The model under review builds one solid part; all positions refer to its coordinate system, in mm. Coordinates: 2 decimals unless noted, no trailing zeros. Order: outer loops, then holes, each group sorted by start corner. A loop starts at its lowest first (then second) coordinate and runs counter-clockwise, first axis right, second up. Notation, with made-up numbers: M 51.25,-6.5 L 81.25,-6.5 A26 ccw 81.25,7.5 Z; hole C -6,-38.75 d10. An arc over 180 degrees is marked long. One line per item, written item: value.
```python
from build123d import *

# Parameters (mm, degrees)
SKETCH1_R           = 5
SKETCH1_R_2         = 1.75
BOSS_EXTRUDE2_DEPTH = 8.5
BOSS_EXTRUDE3_START = -8.5
BOSS_EXTRUDE3_DEPTH = 8.5


with BuildPart() as part:
    # Sketch1 → Boss-Extrude2 (new body)
    # profile 1 of 3: a face of its own
    with BuildSketch(Plane(origin=(0, 0, 0), x_dir=(1, 0, 0), z_dir=(0, 1, 0))):
        Circle(SKETCH1_R)
        with Locations(Location((0, 0, 0), (0, 0, 270))):
            Circle(SKETCH1_R_2, mode=Mode.SUBTRACT)
    # profile 2 of 3: a face of its own
    with BuildSketch(Plane(origin=(0, 0, 0), x_dir=(1, 0, 0), z_dir=(0, 1, 0))):
        with Locations((22, 0)):
            Circle(SKETCH1_R)
        with Locations(Location((22, 0, 0), (0, 0, 270))):
            Circle(SKETCH1_R_2, mode=Mode.SUBTRACT)
    # profile 3 of 3: a face of its own
    with BuildSketch(Plane(origin=(0, 0, 0), x_dir=(1, 0, 0), z_dir=(0, 1, 0))):
        with BuildLine():
            Line((0, 5), (22, 5))
            ThreePointArc((22, 5), (17, 0), (22, -5))
            Line((22, -5), (0, -5))
            ThreePointArc((0, -5), (5, 0), (0, 5))
        make_face()
    extrude(amount=BOSS_EXTRUDE2_DEPTH)

    # Sketch2 → Boss-Extrude3 (add)
    with BuildSketch(Plane(origin=(0, 8.5, 0), x_dir=(1, 0, 0), z_dir=(0, 1, 0)).offset(BOSS_EXTRUDE3_START)):
        with BuildLine():
            Line((22, -5), (25.346400572, -5))
            Line((25.346400572, -5), (31.061757845, -2.212434003))
            add(Edge.make_bspline(
                [(31.061757845, -2.212434003), (38.992757935, 8.50475737), (52.869115173, 6)],
                knots=[0, 0, 0, 1, 1, 1], degree=2))
            Line((52.869115173, 6), (60.222476385, 9.150885415))
            Line((60.222476385, 9.150885415), (58.75, 12.87))
            add(Edge.make_bspline(
                [(11, 5), (27.543585327, 6.057362318), (40.764199153, 18.426668213), (58.75, 12.87)],
                knots=[0, 0, 0, 0, 1, 1, 1, 1], degree=3))
            Line((11, 5), (22, 5))
            ThreePointArc((22, 5), (27, 0), (22, -5))
        make_face()
    extrude(amount=BOSS_EXTRUDE3_DEPTH)


solid = part.part
```
(1) For L1, parallel to X at y = 7.25, z = 0.25; L2, parallel to X at y = 2.25, z = 0; L3, parallel to X at y = 8.25, z = 3, list the stretches that pass through material, from the lowest coordinate up.
Geometry results:
L1: x = -4.99 to -1.73, 1.73 to 20.27, 23.73 to 32.66
L2: x = -5 to -1.75, 1.75 to 20.25, 23.75 to 32.89
L3: x = -4 to 29.45
(2) Mouldability with a two-part tool opening along Z and no side actions: class faces 1 (the cylindrical face through (23.735, 4.19, -0.228)), 2 (the cylindrical face through (-1.71, 4.19, -0.38)), 3 (the flat face through (28.164, 4.19, 3.626)), 4 (the flat face through (5, 4, -5)) as +Z half, -Z half, draft (parallel to the pull), parting line (faces both ways), or undercut.
Geometry results:
face 1: undercut
face 2: undercut
face 3: +Z half
face 4: -Z half
(3) We need section A-A, the plane x = 1. State the section outline as (y, z) points.
Geometry results:
outline: M 0,-5 L 8.5,-5 L 8.5,-1.44 L 0,-1.44 Z; M 0,1.44 L 8.5,1.44 L 8.5,5 L 0,5 Z
(4) We need section B-B, the plane y = 4. Count the separate pieces of the cut face and the enclosed holes in it, plus the area to 3 significant figures.
Geometry results:
separate pieces: 1
enclosed holes: 2
area: 594 mm2
(5) Insertion check: pin 1 Ø2.5 at (x, y) = (3.5, 4.5) entering from -Z; pin 2 Ø2 at (y, z) = (2.5, -8.5) entering from +X. Each pin has a flat end and moves straight along its axis. Give the tip position at first contact, or say it passes through.
Geometry results:
pin 1: stops at z = -5
pin 2: stops at x = 60.22
